Geometry: final body of the model. Coordinates: model frame, mm. Round coordinates to 2 decimals unless told otherwise and drop trailing zeros. Write each loop counter-clockwise with the first axis right and the second up, starting at its lowest first coordinate (ties: lowest second). Pieces come first, ordered by that corner, then holes. Notation, with made-up numbers: M 38,-5 L 61,-5 A23 cw 61,32 Z; hole C 66,37 d3. An arc over 180 degrees is marked long. Use one line per item in the form item = value. Start each with the question number.
Item 1: Ray query, probe 1 along Y at (x, z) = (10, 123); probe 2 along Z at (x, y) = (11, -430). Return the intervals inside material, ascending.
Item 2: Section query B-B (y = -229.5). Return loops of the section in (x, z), and give its area (3 significant figures).
Item 3: Pull-direction query (Y, two-part tool) for faces 1 (the flat face through (6, 0, 71)), 2 (the flat face through (12, -266, 75)), 3 (the flat face through (6, -271, 7)); classes: pulls with the +Y half, pulls with the -Y half, needs draft (parallel to the pull), parting line crosses it, or undercut.
Item 4: Section query A-A (x = 10). Return loops of the section in (y, z).
from build123d import *

# Parameters (mm, degrees)
F0_W     = 12
F0_H     = 140
F1_DEPTH = 540
F2_W     = 6
F2_H     = 6
F3_DEPTH = 140.001
F4_W     = 6
F4_H     = 6
F5_DEPTH = 540.001


with BuildPart() as f1:
    # F0 (on Front) → F1 (new body)
    with BuildSketch(Plane.XZ):
        with Locations((6, 70)):
            Rectangle(F0_W, F0_H)
    extrude(amount=F1_DEPTH)

    # F2 (on Top) → F3 (cut, through all)
    with BuildSketch(Plane.XY):
        with Locations((9, -9)):
            Rectangle(F2_W, F2_H)
        with Locations((9, -531)):
            Rectangle(F2_W, F2_H)
    extrude(amount=F3_DEPTH, mode=Mode.SUBTRACT)

    # F4 (on face) → F5 (cut, through all)
    with BuildSketch(Plane(origin=(0, 0, 0), x_dir=(-1, 0, 0), z_dir=(0, 1, 0))):
        with Locations((-9, 9)):
            Rectangle(F4_W, F4_H)
    extrude(amount=-F5_DEPTH, mode=Mode.SUBTRACT)


solid = f1.part
Working result:
q1.probe_1 = -540 to -534, -528 to -12, -6 to 0
q1.probe_2 = 0 to 6, 12 to 140
q2.outline = M 0,0 L 12,0 L 12,6 L 6,6 L 6,12 L 12,12 L 12,140 L 0,140 Z
q2.area = 1,640 mm²
q3.face_1 = pulls with the +Y half
q3.face_2 = needs draft
q3.face_3 = undercut
q4.outline = M -540,0 L -534,0 L -534,6 L -540,6 Z; M -540,12 L -534,12 L -534,140 L -540,140 Z; M -528,0 L -12,0 L -12,6 L -528,6 Z; M -528,12 L -12,12 L -12,140 L -528,140 Z; M -6,0 L 0,0 L 0,6 L -6,6 Z; M -6,12 L 0,12 L 0,140 L -6,140 Z
